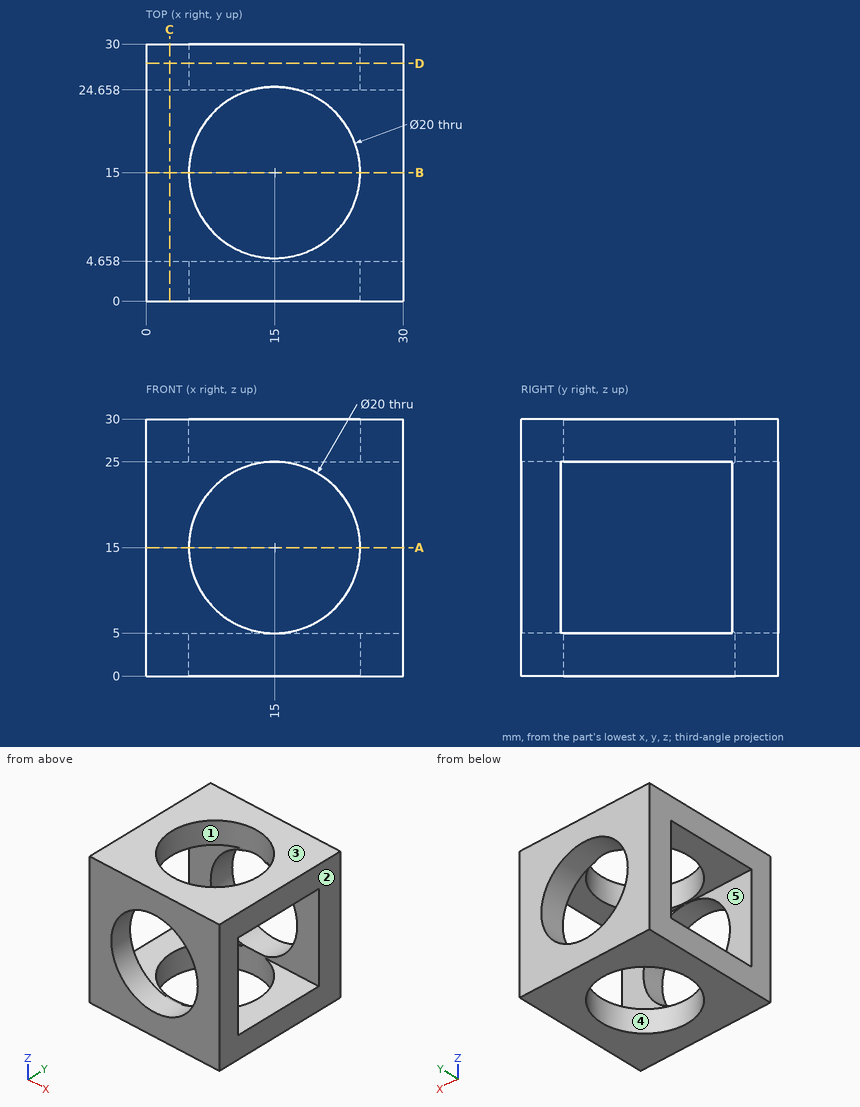
Here's the drawing with two shaded views (mm, measured from the low corner). I have some questions. A direction names the side the tool comes from. Coordinates: 2 decimals unless noted, no trailing zeros. Write each loop counter-clockwise with the first axis right and the second up, starting at its lowest first coordinate (ties: lowest second). Pieces come first, ordered by that corner, then holes. Notation, with made-up numbers: M 87.5,8 L 101.5,8 A21 cw 101.5,42 Z; hole C 13,79.5 d4. An arc over 180 degrees is marked long. Answer as CSV lines item,"result". Start each with the question number.
1) I want a section at D-D, the plane y = 27.75. Please give me the cut outline in (x, z).
2) Please list where these lines run through material, in increasing order: line 1 (Y direction, x = 27, z = 13); line 2 (Z direction, x = 28.75, y = 15.75). Write a range as from..to.
3) We'd pull the mould along X, two halves only. Please class the marked faces 1, 2 and 3: +X half, -X half, draft (parallel to the pull), parting line (faces both ways), or undercut.
4) I want a section at A-A, the plane z = 15. Please give me the cut outline in (x, y), and give its area (3 significant figures).
5) For the marked faces 4 and 5, which set-ups out of +Z, -Z, +X, -X, +Y, -Y let a thin tool reach every point of the face, with its end or its side?
6) I want a section at C-C, the plane x = 2.75. Please give me the cut outline in (y, z).
7) I want a section at B-B, the plane y = 15. Please give me the cut outline in (x, z), and give its area (3 significant figures).
8) For P1, Ø2, axis at y = 12.5, z = 26, coming from the -X side, with a flat end and sliding along its axis, tell me the tip position at first contact or that it passes through.
Data:
1,outline,"M 0,0 L 30,0 L 30,30 L 0,30 Z; hole C 15,15 d20"
2,line 1,"y = 0..4.66, 24.66..30"
2,line 2,"z = 0..5, 25..30"
3,face 1,"undercut"
3,face 2,"+X half"
3,face 3,"draft"
4,outline,"M 0,0 L 5,0 L 5,4.66 L 0,4.66 Z; M 0,24.66 L 5,24.66 L 5,30 L 0,30 Z; M 25,0 L 30,0 L 30,4.66 L 25,4.66 Z; M 25,24.66 L 30,24.66 L 30,30 L 25,30 Z"
4,area,"100 mm^2"
5,face 4,"+Z, -Z"
5,face 5,"+X, -X"
6,outline,"M 0,0 L 30,0 L 30,30 L 0,30 Z; hole M 4.66,5 L 24.66,5 L 24.66,25 L 4.66,25 Z"
7,outline,"M 0,0 L 5,0 L 5,5 L 0,5 Z; M 0,25 L 5,25 L 5,30 L 0,30 Z; M 25,0 L 30,0 L 30,5 L 25,5 Z; M 25,25 L 30,25 L 30,30 L 25,30 Z"
7,area,"100 mm^2"
8,P1,"stops at x = 0"
